Part model, mm, in its own coordinate system. A direction names the side the tool comes from. Round coordinates to 2 decimals unless told otherwise and drop trailing zeros. Write each loop counter-clockwise with the first axis right and the second up, starting at its lowest first coordinate (ties: lowest second). Pieces come first, ordered by that corner, then holes. Notation, with made-up numbers: M 67.5,9 L 98.5,9 A19 cw 98.5,42 Z; hole C -13,19.5 d9. An arc over 180 degrees is marked long. One line per question, with ' | ' between items. Start each with the question number.
1) Saw through at B-B (x = -1). List the corners of the cut face in (y, z).
2) Wall check: probe 1 along Z at (x, y) = (-4, 7.75); probe 2 along X at (y, z) = (0.75, 0). Give the ranges that are in metal, low to high. Write a range as [from, to].
3) Saw through at C-C (y = 9.25). List the corners of the cut face in (x, z).
4) Saw through at A-A (z = 1). List the corners of the cut face in (x, y), plus the area to 3 significant figures.
5) Mould opens along Z. For faces 1 (the face through (6.5, 5, 0)), 2 (the face through (0, 5, -3.75)), 3 (the face through (0, 6, -2.75)), 4 (the face through (2.2, 1, -2.2)) say: pulls with the +Z half, pulls with the -Z half, needs draft (parallel to the pull), parting line crosses it, or undercut.
6) Tool access for faces 5 (the face through (2.1, 1, 2.2)), 6 (the face through (-6.5, 5, 0)): list every direction of +Z, -Z, +X, -X, +Y, -Y with a clear straight run to the whole face (end or side of a thin tool).
7) Saw through at D-D (x = 4.75). List the corners of the cut face in (y, z).
```python
from build123d import *

# Parameters (mm, degrees)
SKETCH1_W           = 13
SKETCH1_H           = 7.5
SKETCH1_W_2         = 11
SKETCH1_H_2         = 5.5
BOSS_EXTRUDE1_DEPTH = 10
SKETCH2_W           = 13
SKETCH2_H           = 7.5
SKETCH2_R           = 2.75
BOSS_EXTRUDE2_DEPTH = 1
BOSS_EXTRUDE3_DEPTH = 3


with BuildPart() as part:
    # Sketch1 → Boss-Extrude1 (new body)
    with BuildSketch(Plane(origin=(0, 0, 0), x_dir=(1, 0, 0), z_dir=(0, 1, 0))):
        Rectangle(SKETCH1_W, SKETCH1_H)
        Rectangle(SKETCH1_W_2, SKETCH1_H_2, mode=Mode.SUBTRACT)
    extrude(amount=BOSS_EXTRUDE1_DEPTH)

    # Sketch2 → Boss-Extrude2 (add)
    with BuildSketch(Plane.XZ):
        Rectangle(SKETCH2_W, SKETCH2_H)
        Circle(SKETCH2_R, mode=Mode.SUBTRACT)
    extrude(amount=-BOSS_EXTRUDE2_DEPTH)

    # Sketch4 → Boss-Extrude3 (add, symmetric)
    with BuildSketch(Plane.XY):
        Polygon((-5.5, 10), (-2.75, 1), (-5.5, 1), align=None)
        Polygon((5.5, 10), (2.75, 1), (5.5, 1), align=None)
    extrude(amount=BOSS_EXTRUDE3_DEPTH, both=True)


solid = part.part
```
Answer key:
1) outline: M 0,-3.75 L 10,-3.75 L 10,-2.75 L 1,-2.75 L 1,-2.56 L 0,-2.56 Z; M 0,2.56 L 1,2.56 L 1,2.75 L 10,2.75 L 10,3.75 L 0,3.75 Z
2) probe 1: z = [-3.75, -2.75], [2.75, 3.75] | probe 2: x = [-6.5, -2.75], [2.75, 6.5]
3) outline: M -6.5,-3.75 L 6.5,-3.75 L 6.5,3.75 L -6.5,3.75 Z; hole M -5.27,-2.75 L 5.27,-2.75 L 5.27,2.75 L -5.27,2.75 Z
4) outline: M -6.5,0 L -2.56,0 L -2.56,1 L -2.75,1 L -5.5,10 L -6.5,10 Z; M 2.56,0 L 6.5,0 L 6.5,10 L 5.5,10 L 2.75,1 L 2.56,1 Z | area: 50.6 mm2
5) face 1: needs draft | face 2: pulls with the -Z half | face 3: undercut | face 4: undercut
6) face 5: +Y | face 6: +Z, -Z, -X, +Y, -Y
7) outline: M 0,-3.75 L 10,-3.75 L 10,-2.75 L 7.55,-2.75 L 7.55,2.75 L 10,2.75 L 10,3.75 L 0,3.75 Z
